Autodesk Inventor part; units mm, degrees
ref_plane "YZ Plane" through (0, 0, 0) normal (1, 0, 0) x (0, 1, 0)
ref_plane "XZ Plane" through (0, 0, 0) normal (0, 1, 0) x (-1, 0, 0)
ref_plane "XY Plane" through (0, 0, 0) normal (0, 0, 1) x (1, 0, 0)
sketch "Sketch1" plane through (0, 0, 0) normal (0, 0, 1) x (1, 0, 0)
  line L0 (0, 20) -> (5, 20)
  line L1 (4, 35) -> (5, 20)
  line L2 (1, 35) -> (0, 20)
  line L3 (1, 35) -> (4, 35)
  point P0 (0, 0)
  dimension "d1" = 5
coil "Coil1" sketch "Sketch1" operation add axis through (-10, 0, 0) along (1, 0, 0) pitch 30 turns 3 hand left
sketch "Sketch2" plane through (0, 0, 0) normal (1, 0, 0) x (0, 1, 0)
  circle A0 centre (0, 0) radius 20
  point P0 (20, 0)
extrude "Extrusion1" add sketch "Sketch2" along normal blind 95
properties part number "rollers"
Design review of the part built by this model. Coordinates are the model's own, in mm. A direction names the side the tool comes from. Coordinates: 2 decimals unless noted, no trailing zeros.
1) Wall thickness on line 1 along X through (y, z) = (-26, 11); line 2 along X through (y, z) = (21.5, 11); line 3 along Y through (x, z) = (81, -1): over which ranges is each line inside the solid? List them lowest first.
2) Take a section at A-A, the plane y = 31.5. State how many separate pieces and enclosed holes the cut face has, and give its area (3 significant figures).
3) For faces 1 (the flat face through (92, 27, 0)), 2 (the flat face through (95, 0, 0)), 3 (the flat face through (2, 27, 0)), list the 3-axis set-ups (+Z, -Z, +X, -X, +Y, -Y) from which the entire face can be reached by the end or side of a thin tool; tool diameter is ignored.
4) Clearance check with flat-ended pins moving along their axes: pin 1 (5 mm diameter, centred on x = 24.5, y = 0.5, fed in from -Z); pin 2 (2 mm diameter, centred on x = 84, z = -22.5, fed in from -Y); pin 3 (2 mm diameter, centred on y = -22, z = -15.5, fed in from +X); pin 4 (4 mm diameter, centred on y = -17, z = -18, fed in from +X). State where each tip first meets the part, or that it passes through.
Returned:
1. line 1: x = 17.46 to 21.36, 47.46 to 51.36, 77.46 to 81.36
1. line 2: x = 28.02 to 32.47, 58.02 to 62.47, 88.02 to 92.47
1. line 3: y = -19.97 to 19.97
2. separate pieces: 4
2. enclosed holes: 0
2. area: 303 mm2
3. face 1: -Z, +X, +Y
3. face 2: +Z, -Z, +X, +Y, -Y
3. face 3: +Z, -X, +Y
4. pin 1: stops at z = -20
4. pin 2: passes through
4. pin 3: stops at x = 76.8
4. pin 4: stops at x = 76.21
